```python
from build123d import *


with BuildPart() as part:
    # Sketch4 → Revolve1 (revolve)
    with BuildSketch(Plane(origin=(0, 0, 0), x_dir=(0, 0, -1), z_dir=(1, 0, 0))):
        with BuildLine():
            Line((0, 0), (-34.925, 0))
            ThreePointArc((-34.925, 0), (-43.905256121, 3.719743879), (-47.625, 12.7))
            Line((-47.625, 12.7), (-47.625, 155.575))
            ThreePointArc((-47.625, 155.575), (-43.905256121, 164.555256121), (-34.925, 168.275))
            Line((-34.925, 168.275), (-31.75, 168.275))
            Line((-31.75, 168.275), (-31.75, 170.188405715))
            Line((-31.75, 170.188405715), (-29.850831966, 170.188405715))
            Line((-29.850831966, 170.188405715), (-29.850831966, 174.113488189))
            Line((-29.850831966, 174.113488189), (-31.75, 174.113488189))
            Line((-31.75, 174.113488189), (-31.75, 176.015383727))
            Line((-31.75, 176.015383727), (-35.259086236, 176.015383727))
            Line((-35.259086236, 176.015383727), (-32.54375, 178.87031185))
            Line((-32.54375, 178.87031185), (-32.54375, 200.025))
            ThreePointArc((-32.54375, 200.025), (-30.683878061, 204.515128061), (-26.19375, 206.375))
            Line((-26.19375, 206.375), (0, 206.375))
            Line((0, 206.375), (0, 0))
        make_face()
    revolve(axis=Axis((0, -30.534688995, 0), (0, 1, 0)))


solid = part.part
```
Geometry: final body of the model. Coordinates: model frame, mm. A direction names the side the tool comes from. Coordinates: 2 decimals unless noted, no trailing zeros. Order: outer loops, then holes, each group sorted by start corner. A loop starts at its lowest first (then second) coordinate and runs counter-clockwise, first axis right, second up. Notation, with made-up numbers: M 56,71 L 76,71 A7 ccw 76,83 Z; hole C -22.5,-14.5 d2. An arc over 180 degrees is marked long. Answer as CSV lines item,"result".
Q1. Section B-B on z = 0. Return the cut outline in (x, y) (3 decimals), and give its area (3 significant figures).
Answers:
outline,"M -47.625,12.7 A12.7 ccw -34.925,0 L 34.925,0 A12.7 ccw 47.625,12.7 L 47.625,155.575 A12.7 ccw 34.925,168.275 L 31.75,168.275 L 31.75,170.188 L 29.851,170.188 L 29.851,174.113 L 31.75,174.113 L 31.75,176.015 L 35.259,176.015 L 32.544,178.87 L 32.544,200.025 A6.35 ccw 26.194,206.375 L -26.194,206.375 A6.35 ccw -32.544,200.025 L -32.544,178.87 L -35.259,176.015 L -31.75,176.015 L -31.75,174.113 L -29.851,174.113 L -29.851,170.188 L -31.75,170.188 L -31.75,168.275 L -34.925,168.275 A12.7 ccw -47.625,155.575 Z"
area,"18,300 mm^2"
Q2. Section C-C on y = 73. Return the cut outline in (x, z) (3 decimals).
Answers:
outline,"C 0,0 d95.25"
Q3. Draft query along Y for faces 3 (the conical face through (1.437, 178.732, -32.644)), 4 (the flat face through (5, 176.015, 32)), 5 (the flat face through (0, 0, 0)), 6 (the cylindrical face through (-19.802, 189.596, -25.826)). Return one class per face: pulls with the +Y half, pulls with the -Y half, needs draft (parallel to the pull), parting line crosses it, or undercut.
Answers:
face 3,"pulls with the +Y half"
face 4,"undercut"
face 5,"pulls with the -Y half"
face 6,"needs draft"
Q4. Set-up query: faces 1 (the cylindrical face through (29.597, 172.178, -3.886)), 2 (the flat face through (0, 206.375, 0)). Return all of +Z, -Z, +X, -X, +Y, -Y with unobstructed straight access to the full face (end or side cutting, diameter ignored); none if empty.
Answers:
face 1,"none"
face 2,"+Z, -Z, +X, -X, +Y"
Q5. Section A-A on x = 0. Return the cut outline in (y, z) (3 decimals), and give its area (3 significant figures).
Answers:
outline,"M 0,-34.925 A12.7 ccw 12.7,-47.625 L 155.575,-47.625 A12.7 ccw 168.275,-34.925 L 168.275,-31.75 L 170.188,-31.75 L 170.188,-29.851 L 174.113,-29.851 L 174.113,-31.75 L 176.015,-31.75 L 176.015,-35.259 L 178.87,-32.544 L 200.025,-32.544 A6.35 ccw 206.375,-26.194 L 206.375,26.194 A6.35 ccw 200.025,32.544 L 178.87,32.544 L 176.015,35.259 L 176.015,31.75 L 174.113,31.75 L 174.113,29.851 L 170.188,29.851 L 170.188,31.75 L 168.275,31.75 L 168.275,34.925 A12.7 ccw 155.575,47.625 L 12.7,47.625 A12.7 ccw 0,34.925 Z"
area,"18,300 mm^2"
Q6. Line query: probe 1 along X at (y, z) = (47.5, 32); probe 2 along X at (y, z) = (166.5, -25.5); probe 3 along Y at (x, z) = (-24, 24.5) (3 decimals). Output: solid intervals per line, ascending. Write a range as [from, to].
Answers:
probe 1,"x = [-35.27, 35.27]"
probe 2,"x = [-32.62, 32.62]"
probe 3,"y = [0, 168.275], [176.015, 177.027]"
Q7. First-contact query: P1, Ø4, axis at y = 69.5, z = 16, coming from the +X side; P2, Ø12, axis at x = 23, z = -23.5, coming from the +Y side; P3, Ø3, axis at x = -2, y = 136.5, coming from the +Z side. Flat tips, straight axial feed; report the tip coordinate or a pass-through.
Answers:
P1,"stops at x = 45.52"
P2,"stops at y = 206.34"
P3,"stops at z = 47.62"
